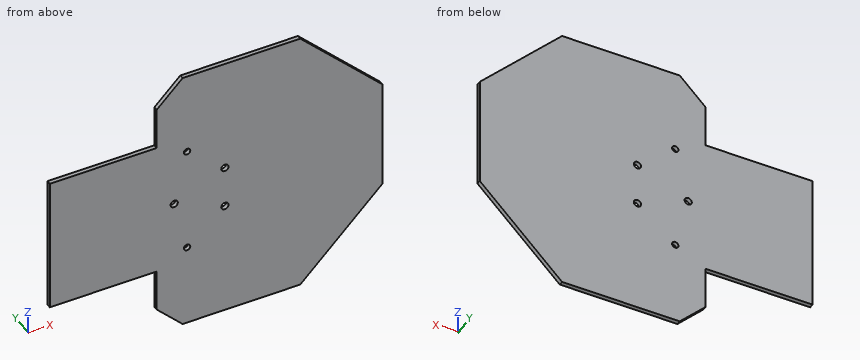
from build123d import *

# Parameters (mm, degrees)
BOSS_EXTRUDE1_DEPTH = 2
SKETCH2_R           = 1.7
CUT_EXTRUDE1_DEPTH  = 167.639739727
CUT_EXTRUDE2_REACH  = 168.64
SKETCH7_R           = 1.5
SKETCH10_W          = 64.75
SKETCH10_H          = 2
BOSS_EXTRUDE3_DEPTH = 50


with BuildPart() as part:
    # Sketch1 → Boss-Extrude1 (new body)
    with BuildSketch(Plane(origin=(0, 0, 0), x_dir=(1, 0, 0), z_dir=(0, 1, 0))):
        Polygon((0, 12.09), (0, 116.84), (12.09, 128.93), (67.09, 128.93), (105.554999675, 90.46), (105.554999675, 38.46), (67.09, 0), (12.09, 0), align=None)
    extrude(amount=BOSS_EXTRUDE1_DEPTH)

    # Sketch2 → Cut-Extrude1 (cut, through all)
    with BuildSketch(Plane(origin=(0, 2, 0), x_dir=(1, 0, 0), z_dir=(0, 1, 0))):
        with Locations(Location((8.15, 64.465, 0), (0, 0, 270))):
            Circle(SKETCH2_R)
        with Locations(Location((31.85, 54.465, 0), (0, 0, 270))):
            Circle(SKETCH2_R)
        with Locations(Location((31.85, 74.465, 0), (0, 0, 270))):
            Circle(SKETCH2_R)
    extrude(amount=-CUT_EXTRUDE1_DEPTH, mode=Mode.SUBTRACT)

    # Sketch7 → Cut-Extrude2 (cut, up to next)
    with BuildSketch(Plane(origin=(0, 2, 0), x_dir=(1, 0, 0), z_dir=(0, 1, 0)), mode=Mode.PRIVATE) as cut_extrude2_sk1:
        with Locations(Location((14.18, 89.57, 0), (0, 0, 270))):
            Circle(SKETCH7_R)
    cut_extrude2_tool1 = extrude(cut_extrude2_sk1.sketch, amount=-CUT_EXTRUDE2_REACH, mode=Mode.PRIVATE) & part.part
    # Sketch7 → Cut-Extrude2 (cut, up to next)
    with BuildSketch(Plane(origin=(0, 2, 0), x_dir=(1, 0, 0), z_dir=(0, 1, 0)), mode=Mode.PRIVATE) as cut_extrude2_sk2:
        with Locations(Location((14.177621555, 39.358656737, 0), (0, 0, 90))):
            Circle(SKETCH7_R)
    cut_extrude2_tool2 = extrude(cut_extrude2_sk2.sketch, amount=-CUT_EXTRUDE2_REACH, mode=Mode.PRIVATE) & part.part
    add(cut_extrude2_tool1.solids().sort_by_distance((14.18, 2, -89.57))[0], mode=Mode.SUBTRACT)
    add(cut_extrude2_tool2.solids().sort_by_distance((14.177622, 2, -39.358657))[0], mode=Mode.SUBTRACT)

    # Sketch10 → Boss-Extrude3 (add)
    with BuildSketch(Plane.ZY):
        with Locations((-64.465, 1)):
            Rectangle(SKETCH10_W, SKETCH10_H)
    extrude(amount=BOSS_EXTRUDE3_DEPTH)


solid = part.part
Geometry check sheet. Reference: the model listing, model coordinates, mm. Round coordinates to 2 decimals unless told otherwise and drop trailing zeros. Write each loop counter-clockwise with the first axis right and the second up, starting at its lowest first coordinate (ties: lowest second). Pieces come first, ordered by that corner, then holes. Notation, with made-up numbers: (-29, 65) - (-13, 65) arc R7 cw to (-13, 74) - close; hole circle Ø5 at (68.5, -27). An arc over 180 degrees is marked (long way). One line per item, written item: value.
1. Cross-section at C-C on y = 0.4. Record the boundary of the cut face in (x, z) (3 decimals).
The answers:
outline: (-50, -96.84) - (0, -96.84) - (0, -116.84) - (12.09, -128.93) - (67.09, -128.93) - (105.555, -90.46) - (105.555, -38.46) - (67.09, 0) - (12.09, 0) - (0, -12.09) - (0, -32.09) - (-50, -32.09) - close; hole circle Ø3.4 at (8.15, -64.465); hole circle Ø3 at (14.178, -39.359); hole circle Ø3 at (14.18, -89.57); hole circle Ø3.4 at (31.85, -74.465); hole circle Ø3.4 at (31.85, -54.465)
2. Cross-section at D-D on z = -16. Record the boundary of the cut face in (x, y), and give its area (3 significant figures).
The answers:
outline: (0, 0) - (83.09, 0) - (83.09, 2) - (0, 2) - close
area: 166 mm^2
3. Depth check by flat-ended pin: pin 1 Ø3 at (x, z) = (31.85, -54.465) entering from -Y; pin 2 Ø0.6 at (y, z) = (0.5, -25.5) entering from -X. Enter the tip coordinate at first touch or a pass-through.
The answers:
pin 1: passes through
pin 2: stops at x = 0
4. Scan lines: L1, parallel to X at y = 1, z = -89.57 (3 decimals); L2, parallel to Z at x = -11, y = 0.2; L3, parallel to Z at x = 30.5, y = 0.35. Record each from-to range of solid material in increasing order.
The answers:
L1: x = -50 to 12.68, 15.68 to 105.555
L2: z = -96.84 to -32.09
L3: z = -128.93 to -75.5, -73.43 to -55.5, -53.43 to 0
5. Cross-section at B-B on x = 8.15. Record the boundary of the cut face in (y, z) (3 decimals).
The answers:
outline: (0, -124.99) - (2, -124.99) - (2, -66.165) - (0, -66.165) - close; (0, -62.765) - (2, -62.765) - (2, -3.94) - (0, -3.94) - close
6. Cross-section at A-A on x = 31.85. Record the boundary of the cut face in (y, z) (3 decimals), and give its area (3 significant figures).
The answers:
outline: (0, -128.93) - (2, -128.93) - (2, -76.165) - (0, -76.165) - close; (0, -72.765) - (2, -72.765) - (2, -56.165) - (0, -56.165) - close; (0, -52.765) - (2, -52.765) - (2, 0) - (0, 0) - close
area: 244 mm^2
